```python
from build123d import *

# Parameters (mm, degrees)
SKETCH_1_R               = 10
SKETCH_1_R_2             = 2.5
EXTRUDE_1_DEPTH          = 70
SKETCH_2_W               = 60
SKETCH_2_H               = 70
SKETCH_2_H_2             = 67.94057246
CUT_EXTRUDE_1_DEPTH      = 70
EXTRUDE_2_DEPTH          = 60
EXTRUDE_3_DEPTH          = 60
CUT_EXTRUDE_3_DEPTH      = 129.790186287
CUT_EXTRUDE_3_DEPTH_BACK = 129.790186287
SKETCH_6_R               = 2.5
CUT_EXTRUDE_4_DEPTH      = 132.384596068
CUT_EXTRUDE_4_DEPTH_BACK = 132.384596068
SKETCH_7_W               = 41.69897569
SKETCH_7_H               = 124.994220232
SKETCH_7_W_2             = 29.374155289
SKETCH_7_H_2             = 127.870011659
CUT_EXTRUDE_5_DEPTH      = 99.780560832
CUT_EXTRUDE_5_DEPTH_BACK = 99.780560832
SKETCH_9_R               = 2.5
EXTRUDE_4_DEPTH          = 2


with BuildPart() as part:
    # Sketch 1 → Extrude 1 (new body)
    with BuildSketch(Plane.XY):
        with BuildLine():
            Line((-15, 90), (-15, 0))
            ThreePointArc((-15, 0), (0, -15), (15, 0))
            Line((15, 0), (15, 90))
            ThreePointArc((15, 90), (0, 105), (-15, 90))
        make_face()
        Circle(SKETCH_1_R, mode=Mode.SUBTRACT)
        with Locations((0, 90)):
            Circle(SKETCH_1_R_2, mode=Mode.SUBTRACT)
    extrude(amount=EXTRUDE_1_DEPTH)

    # Sketch 2 → Cut-Extrude 1 (cut)
    with BuildSketch(Plane.ZY.offset(15)):
        with Locations((35, 80)):
            Rectangle(SKETCH_2_W, SKETCH_2_H)
        with Locations((35, 11.02971377)):
            Rectangle(SKETCH_2_W, SKETCH_2_H_2)
    extrude(amount=-CUT_EXTRUDE_1_DEPTH, mode=Mode.SUBTRACT)


with BuildPart() as cut_extrude_1_piece_1:
    # of the separate pieces the step leaves, piece 1, a body of its own (cut_extrude_1_pieces)
    add(part.part.solids().sort_by_distance((15, 0, 0))[0])



with BuildPart() as cut_extrude_1_piece_2:
    # of the separate pieces the step leaves, piece 2, a body of its own (cut_extrude_1_pieces)
    add(part.part.solids().sort_by_distance((15, 0, 65))[0])


with BuildPart() as cut_extrude_1_piece_1_1:
    add(cut_extrude_1_piece_1.part)

    add(cut_extrude_1_piece_2.part)  # Extrude 2 merges Cut-Extrude 1 piece 2
    # Sketch 4 → Extrude 2 (add)
    with BuildSketch(Plane(origin=(0, 0, 65), x_dir=(-1, 0, 0), z_dir=(0, 0, -1))):
        with BuildLine():
            Line((-4.490156776, 68.758657712), (15, 57.50601045))
            Line((15, 57.50601045), (36.319312502, 12.911360415))
            ThreePointArc((36.319312502, 12.911360415), (35.142094618, 9.577570071), (31.808304274, 10.754787955))
            Line((31.808304274, 10.754787955), (15, 45.913541163))
            Line((15, 45.913541163), (-9.509843224, 60.064305746))
            ThreePointArc((-9.509843224, 60.064305746), (-11.347175983, 66.921324953), (-4.490156776, 68.758657712))
        make_face()
    extrude(amount=EXTRUDE_2_DEPTH)

    # Sketch 5 → Extrude 3 (add)
    with BuildSketch(Plane(origin=(0, 0, 65), x_dir=(-1, 0, 0), z_dir=(0, 0, -1))):
        with BuildLine():
            Line((-30.017605928, 49.094069219), (-15, 60.919508718))
            Line((-15, 60.919508718), (12.5, 45.042376315))
            ThreePointArc((12.5, 45.042376315), (14.330127019, 38.212249296), (7.5, 36.382122277))
            Line((7.5, 36.382122277), (-15, 49.372503334))
            Line((-15, 49.372503334), (-27.615908762, 44.780688066))
            ThreePointArc((-27.615908762, 44.780688066), (-30.655195979, 45.913733224), (-30.017605928, 49.094069219))
        make_face()
    extrude(amount=EXTRUDE_3_DEPTH)

    # Sketch 6 → Cut-Extrude 3 (cut, two sides: drawn at the far end of the back side and taken through both)
    with BuildSketch(Plane(origin=(0, 0, 65), x_dir=(-1, 0, 0), z_dir=(0, 0, -1)).offset(-CUT_EXTRUDE_3_DEPTH_BACK)):
        with Locations(Location((-7, 64.411481729, 0), (0, 0, 90))):
            Circle(SKETCH_6_R)
        with Locations(Location((-11.650635095, 53.212249296, 0), (0, 0, 90))):
            Circle(SKETCH_6_R)
        with Locations(Location((10, 40.712249296, 0), (0, 0, 90))):
            Circle(SKETCH_6_R)
        with Locations(Location((10.320508076, 54.411481729, 0), (0, 0, 90))):
            Circle(SKETCH_6_R)
    extrude(amount=CUT_EXTRUDE_3_DEPTH + CUT_EXTRUDE_3_DEPTH_BACK, mode=Mode.SUBTRACT)

    # Sketch 7 → Cut-Extrude 4 (cut, two sides: drawn at the far end of the back side and taken through both)
    with BuildSketch(Plane(origin=(0, 0, 0), x_dir=(0, 0, -1), z_dir=(1, 0, 0)).offset(-CUT_EXTRUDE_4_DEPTH_BACK)):
        with Locations((15.849487845, 45.30812051)):
            Rectangle(SKETCH_7_W, SKETCH_7_H)
        with Locations((-79.687077644, 43.870224797)):
            Rectangle(SKETCH_7_W_2, SKETCH_7_H_2)
    extrude(amount=CUT_EXTRUDE_4_DEPTH + CUT_EXTRUDE_4_DEPTH_BACK, mode=Mode.SUBTRACT)


with BuildPart() as cut_extrude_4_piece_1:
    # of the separate pieces the step leaves, piece 1, a body of its own (cut_extrude_4_pieces)
    add(cut_extrude_1_piece_1_1.part.solids().sort_by_distance((-15, 45.913541163, 65))[0])

    # Sketch 8 → Cut-Extrude 5 (cut, two sides: drawn at the far end of the back side and taken through both)
    with BuildSketch(Plane(origin=(0, 0, 5), x_dir=(-1, 0, 0), z_dir=(0, 0, -1)).offset(-CUT_EXTRUDE_5_DEPTH_BACK)):
        Polygon((-6.948831874, 74.137409514), (-14.942987604, 67.665950114), (-12.735077926, 60.813816632), (14.064377472, 45.130044439), (31.727654893, 6.225153222), (50.98976346, 4.626322076), (26.322082923, 67.665950114), align=None)
    extrude(amount=CUT_EXTRUDE_5_DEPTH + CUT_EXTRUDE_5_DEPTH_BACK, mode=Mode.SUBTRACT)


with BuildPart() as cut_extrude_4_piece_2:
    # of the separate pieces the step leaves, piece 2, a body of its own (cut_extrude_4_pieces)
    add(cut_extrude_1_piece_1_1.part.solids().sort_by_distance((27.615908762, 44.780688066, 65))[0])

    # Sketch 9 → Extrude 4 (add)
    with BuildSketch(Plane(origin=(0, 0, 5), x_dir=(-1, 0, 0), z_dir=(0, 0, -1))):
        with BuildLine():
            Line((-27.615908762, 44.780688066), (-15, 49.372503334))
            Line((-15, 49.372503334), (7.5, 36.382122277))
            ThreePointArc((7.5, 36.382122277), (14.330127019, 38.212249296), (12.5, 45.042376315))
            Line((12.5, 45.042376315), (-15, 60.919508718))
            Line((-15, 60.919508718), (-30.017605928, 49.094069219))
            ThreePointArc((-30.017605928, 49.094069219), (-30.655195979, 45.913733224), (-27.615908762, 44.780688066))
        make_face()
        with Locations(Location((-11.650635095, 53.212249296, 0), (0, 0, 90))):
            Circle(SKETCH_9_R, mode=Mode.SUBTRACT)
        with Locations(Location((10, 40.712249296, 0), (0, 0, 90))):
            Circle(SKETCH_9_R, mode=Mode.SUBTRACT)
    extrude(amount=EXTRUDE_4_DEPTH)


solid = cut_extrude_4_piece_2.part
```
The listing builds one solid part. Answer for the finished solid, in the listing's coordinates (mm). A direction names the side the tool comes from. Give positions to 0.01 mm unless a question says otherwise; leave off trailing zeros. Order: outer loops, then holes, each group sorted by start corner. A loop starts at its lowest first (then second) coordinate and runs counter-clockwise, first axis right, second up. Notation, with made-up numbers: (79, 21.25) - (96, 21.25) arc R10 cw to (96, 39.25) - close; hole circle Ø9 at (-30, 18). An arc over 180 degrees is marked (long way). Use one line per item in the form item = value. Start each with the question number.
(1) Flat-ended cylindrical pins translate along their axes: pin 1 Ø10 at (y, z) = (39.5, 29.5) entering from +X; pin 2 Ø8 at (x, y) = (18.5, 41.5) entering from +Z; pin 3 Ø3 at (x, z) = (20.5, 28.5) entering from +Y; pin 4 Ø4 at (y, z) = (56.5, 22.5) entering from +X. Find the tip coordinate at first contact, or state that the pin passes through.
(2) A cutting plane is placed at C-C, the plane x = -10. Write down the section's boundary in (y, z).
(3) For faces 4 (the flat face through (3.91, 42.97, 34.43)), 5 (the flat face through (1.06, 52.87, 34.43)), determine the directions among +Z, -Z, +X, -X, +Y, -Y from which every point of the face is accessible in a straight line to the end or side of a thin tool.
(4) A cutting plane is placed at B-B, the plane z = 61.5. Write down the section's boundary in (x, y), then the cut area to 3 significant figures.
(5) A cutting plane is placed at A-A, the plane y = 54.25. Write down the section's boundary in (x, z).
(6) A cutting plane is placed at D-D, the plane y = 59.25. Write down the section's boundary in (x, z).
(7) The mould has two halves that part along Y. Classify faces 1 (the flat face through (8, 48, 65)), 2 (the cylindrical face through (30.7, 46, 34.4)), 3 (the cylindrical face through (9.21, 52.67, 34.43)): released by +Y, released by -Y, zero draft, split by the parting line, or undercut.
(8) Consider line 1 (X direction, y = 40.5, z = 34); line 2 (Y direction, x = -10, z = 51); line 3 (X direction, y = 38.5, z = 25). Determine where each line is inside the solid, lowest interval first. Write a range as from..to.
Ans:
q1.pin_1 = 6.56
q1.pin_2 = through
q1.pin_3 = 57.77
q1.pin_4 = 23.15
q2.outline = (35.71, 3) - (38.21, 3) - (38.21, 65) - (35.71, 65) - close; (43.21, 3) - (46.49, 3) - (46.49, 65) - (43.21, 65) - close
q3.face_4 = +Z, -Z, -Y
q3.face_5 = +Z, -Z, -X, +Y
q4.outline = (-12.5, 45.04) arc R5 ccw to (-7.5, 36.38) - (15, 49.37) - (27.62, 44.78) arc R2.5 ccw to (30.02, 49.09) - (15, 60.92) - close; hole circle Ø5 at (-10, 40.71); hole circle Ø5 at (11.65, 53.21)
q4.area = 416 mm^2
q5.outline = (3.45, 3) - (9.38, 3) - (9.38, 65) - (3.45, 65) - close; (13.93, 3) - (23.47, 3) - (23.47, 65) - (13.93, 65) - close
q6.outline = (12.11, 3) - (17.12, 3) - (17.12, 65) - (12.11, 65) - close
q7.face_1 = zero draft
q7.face_2 = split by the parting line
q7.face_3 = undercut
q8.line_1 = -15..-12.49, -7.51..-0.37
q8.line_2 = 35.71..38.21, 43.21..46.49
q8.line_3 = -14.48..-11.16, -8.84..-3.83
